```python
from build123d import *

# Parameters (mm, degrees)
RURA_KWADRATOWA_30_X_30_X_2_6_1_DEPTH = 60
SZKIC3_R                              = 5
WYTNIJ_WYCI_GNI_CIE1_DEPTH            = 69.738635424


with BuildPart() as part:
    # Sketch11 → Rura kwadratowa 30 X 30 X 2.6(1) (new body)
    with BuildSketch(Plane(origin=(0, 0, 0), x_dir=(0, 0, -1), z_dir=(1, 0, 0))):
        with BuildLine():
            Line((-9.8, -15), (9.8, -15))
            ThreePointArc((9.8, -15), (13.476955262, -13.476955262), (15, -9.8))
            Line((15, -9.8), (15, 9.8))
            ThreePointArc((15, 9.8), (13.476955262, 13.476955262), (9.8, 15))
            Line((9.8, 15), (-9.8, 15))
            ThreePointArc((-9.8, 15), (-13.476955262, 13.476955262), (-15, 9.8))
            Line((-15, 9.8), (-15, -9.8))
            ThreePointArc((-15, -9.8), (-13.476955262, -13.476955262), (-9.8, -15))
        make_face()
        with BuildLine():
            Line((-9.8, -12.4), (9.8, -12.4))
            ThreePointArc((9.8, -12.4), (11.638477631, -11.638477631), (12.4, -9.8))
            Line((12.4, -9.8), (12.4, 9.8))
            ThreePointArc((12.4, 9.8), (11.638477631, 11.638477631), (9.8, 12.4))
            Line((9.8, 12.4), (-9.8, 12.4))
            ThreePointArc((-9.8, 12.4), (-11.638477631, 11.638477631), (-12.4, 9.8))
            Line((-12.4, 9.8), (-12.4, -9.8))
            ThreePointArc((-12.4, -9.8), (-11.638477631, -11.638477631), (-9.8, -12.4))
        make_face(mode=Mode.SUBTRACT)
    extrude(amount=RURA_KWADRATOWA_30_X_30_X_2_6_1_DEPTH)

    # Szkic3 → Wytnij-wyciągnięcie1 (cut, through all)
    with BuildSketch(Plane.XY.offset(15)):
        with Locations(Location((30, 5, 0), (0, 0, 73.739795292))):
            Circle(SZKIC3_R)
    extrude(amount=-WYTNIJ_WYCI_GNI_CIE1_DEPTH, mode=Mode.SUBTRACT)


solid = part.part
```
Model file for the job. Use its own axes, mm. A direction names the side the tool comes from. Give positions to 0.01 mm unless a question says otherwise; leave off trailing zeros. Loops run counter-clockwise (first coordinate to the right, second up) from the corner with the lowest first, then second, coordinate; pieces in that order, holes last. Notation, with made-up numbers: (16.5, 89.5) - (59.5, 89.5) arc R28 ccw to (59.5, 112.5) - close; hole circle Ø3 at (78.25, -21). An arc over 180 degrees is marked (long way). One line per item, written item: value. Start each with the question number.
1. Pull direction Z, two halves, no side cores. Call faces 3 (the cylindrical face through (29.58, 11.618, -11.659)), 4 (the flat face through (0, 0, -13)), 5 (the cylindrical face through (29.58, 13.436, -13.517)): pulls with the +Z half, pulls with the -Z half, needs draft (parallel to the pull), parting line crosses it, or undercut.
2. Pin check, flat tip, straight feed: pin 1 (2 mm diameter, centred on y = 1.5, z = 10.5, fed in from +X). Stop position of the tip, or through.
3. Which spindle directions (+Z, -Z, +X, -X, +Y, -Y) get a long thin tool onto all of the face, cutting with end or side? Do faces 1 (the cylindrical face through (29.58, -11.659, -11.618)), 2 (the cylindrical face through (30, 10, -14)). Say none if no direction does.
4. Slice it at C-C (y = 5). List the corners of the cut face in (x, z), plus the area to 3 significant figures.
5. Probe L1, parallel to Z at x = 18, y = -6; L2, parallel to X at y = 5, z = -13.5. List the from-to ranges inside material, lowest first. Write a range as from..to.
6. Slice it at A-A (y = -3). List the corners of the cut face in (x, z), plus the area to 3 significant figures.
7. Slice it at D-D (x = 20). List the corners of the cut face in (y, z), plus the area to 3 significant figures.
Solution:
1. face 3: undercut
1. face 4: needs draft
1. face 5: pulls with the -Z half
2. pin 1: passes through
3. face 1: +X, -X
3. face 2: +Z, -Z
4. outline: (0, -15) - (25, -15) - (25, -12.4) - (0, -12.4) - close; (0, 12.4) - (25, 12.4) - (25, 15) - (0, 15) - close; (35, -15) - (60, -15) - (60, -12.4) - (35, -12.4) - close; (35, 12.4) - (60, 12.4) - (60, 15) - (35, 15) - close
4. area: 260 mm^2
5. L1: z = -15..-12.4, 12.4..15
5. L2: x = 0..25, 35..60
6. outline: (0, -15) - (60, -15) - (60, -12.4) - (0, -12.4) - close; (0, 12.4) - (60, 12.4) - (60, 15) - (0, 15) - close
6. area: 312 mm^2
7. outline: (-15, -9.8) arc R5.2 ccw to (-9.8, -15) - (9.8, -15) arc R5.2 ccw to (15, -9.8) - (15, 9.8) arc R5.2 ccw to (9.8, 15) - (-9.8, 15) arc R5.2 ccw to (-15, 9.8) - close; hole (-12.4, -9.8) arc R2.6 ccw to (-9.8, -12.4) - (9.8, -12.4) arc R2.6 ccw to (12.4, -9.8) - (12.4, 9.8) arc R2.6 ccw to (9.8, 12.4) - (-9.8, 12.4) arc R2.6 ccw to (-12.4, 9.8) - close
7. area: 268 mm^2
